Autodesk Inventor part; units mm, degrees
ref_plane "C1_XY" through (0, 0, 0) normal (0, 0, 1) x (1, 0, 0)
ref_plane "C1_YZ" through (0, 0, 0) normal (1, 0, 0) x (0, 1, 0)
ref_plane "C1_ZX" through (0, 0, 0) normal (0, 1, 0) x (0, 0, 1)
sketch "Sketch_63" plane through (0, 0, 0) normal (0, 0, 1) x (1, 0, 0)
  line L0 (-10, -3) -> (-10, -9)
  arc A0 (-10, -9) -> (-9, -10) centre (-9, -9) ccw
  line L1 (-9, -10) -> (9, -10)
  arc A1 (9, -10) -> (10, -9) centre (9, -9) ccw
  line L2 (10, -9) -> (10, -3)
  line L3 (10, -3) -> (8, -3)
  line L4 (8, -3) -> (8, -6)
  line L5 (8, -6) -> (7.0607, -6)
  line L6 (7.0607, -6) -> (4, -2.9393)
  line L7 (4, -2.9393) -> (4, -0.5196)
  line L8 (4, -0.5196) -> (3.7, 0)
  line L9 (3.7, 0) -> (4, 0.5196)
  line L10 (4, 0.5196) -> (4, 2.9393)
  line L11 (4, 2.9393) -> (7.0607, 6)
  line L12 (7.0607, 6) -> (8, 6)
  line L13 (8, 6) -> (8, 3)
  line L14 (8, 3) -> (10, 3)
  line L15 (10, 3) -> (10, 9)
  arc A2 (10, 9) -> (9, 10) centre (9, 9) ccw
  line L16 (9, 10) -> (3, 10)
  line L17 (3, 10) -> (3, 8)
  line L18 (3, 8) -> (6, 8)
  line L19 (6, 8) -> (6, 7.0607)
  line L20 (6, 7.0607) -> (2.9393, 4)
  line L21 (2.9393, 4) -> (0.5196, 4)
  line L22 (0.5196, 4) -> (0, 3.7)
  line L23 (0, 3.7) -> (-0.5196, 4)
  line L24 (-0.5196, 4) -> (-2.9393, 4)
  line L25 (-2.9393, 4) -> (-6, 7.0607)
  line L26 (-6, 7.0607) -> (-6, 8)
  line L27 (-6, 8) -> (-3, 8)
  line L28 (-3, 8) -> (-3, 10)
  line L29 (-3, 10) -> (-9, 10)
  arc A3 (-9, 10) -> (-10, 9) centre (-9, 9) ccw
  line L30 (-10, 9) -> (-10, 3)
  line L31 (-10, 3) -> (-8, 3)
  line L32 (-8, 3) -> (-8, 6)
  line L33 (-8, 6) -> (-7.0607, 6)
  line L34 (-7.0607, 6) -> (-4, 2.9393)
  line L35 (-4, 2.9393) -> (-4, 0.5196)
  line L36 (-4, 0.5196) -> (-3.7, 0)
  line L37 (-3.7, 0) -> (-4, -0.5196)
  line L38 (-4, -0.5196) -> (-4, -2.9393)
  line L39 (-4, -2.9393) -> (-7.0607, -6)
  line L40 (-7.0607, -6) -> (-8, -6)
  line L41 (-8, -6) -> (-8, -3)
  line L42 (-8, -3) -> (-10, -3)
  line L43 (-6, -7.2678) -> (-6, -7.5)
  arc A4 (-6, -7.5) -> (-5.5, -8) centre (-5.5, -7.5) ccw
  line L44 (-5.5, -8) -> (5.5, -8)
  arc A5 (5.5, -8) -> (6, -7.5) centre (5.5, -7.5) ccw
  line L45 (6, -7.5) -> (6, -7.2678)
  arc A6 (6, -7.2678) -> (5.8536, -6.9142) centre (5.5, -7.2678) ccw
  line L46 (5.8536, -6.9142) -> (3.0858, -4.1464)
  arc A7 (3.0858, -4.1464) -> (2.7322, -4) centre (2.7322, -4.5) ccw
  line L47 (2.7322, -4) -> (-2.7322, -4)
  arc A8 (-2.7322, -4) -> (-3.0858, -4.1464) centre (-2.7322, -4.5) ccw
  line L48 (-3.0858, -4.1464) -> (-5.8536, -6.9142)
  arc A9 (-5.8536, -6.9142) -> (-6, -7.2678) centre (-5.5, -7.2678) ccw
extrude "Extrusion1" add sketch "Sketch_63" against normal blind 440
sketch "Sketch2" plane through (0, 0, -440) normal (0, 0, -1) x (-1, 0, 0)
  point P0 (0, 0)
hole "Hole1" at (0, 0, -440) direction (0, 0, 1) diameter 4.2 depth 440
ref_plane "C1_XY" through (0, 0, 0) normal (0, 0, 1) x (1, 0, 0)
ref_plane "C1_YZ" through (0, 0, 0) normal (1, 0, 0) x (0, 1, 0)
ref_plane "C1_ZX" through (0, 0, 0) normal (0, 1, 0) x (0, 0, 1)
thread "Thread1"
thread "Thread2"
properties part number "HFSFB5-2020-440" material "Aluminum 6061"
Geometry: final body of the model. Coordinates: model frame, mm. Round coordinates to 2 decimals unless told otherwise and drop trailing zeros. Put each result on its own line as item: value. Start each with the question number.
Q1. Section A-A on z = -194. Give the number of separate pieces and of enclosed holes in the cut face, and give its area (3 significant figures).
Q2. Line query: probe 1 along Y at (x, z) = (4.75, -345); probe 2 along Y at (x, z) = (0, -267.5); probe 3 along X at (y, z) = (0, -94.5). Output: solid intervals per line, ascending.
Q3. First-contact query: pin 1 (2.5 mm diameter, centred on x = 0, y = 0, fed in from -Z); pin 2 (1.2 mm diameter, centred on y = -1.5, z = -324, fed in from +X). Flat tips, straight axial feed; report the tip coordinate or a pass-through.
Q4. Pull-direction query (X, two-part tool) for faces 1 (the flat face through (0, -8, -217)), 2 (the flat face through (-2.4, 0.1, 0)); classes: +X half, -X half, draft (parallel to the pull), parting line (faces both ways), or undercut.
Ans:
1. separate pieces: 1
1. enclosed holes: 2
1. area: 194 mm2
2. probe 1: y = -10 to -8, -5.81 to -3.69, 3.69 to 5.81, 8 to 10
2. probe 2: y = -10 to -8, -4 to -2.1, 2.1 to 3.7
2. probe 3: x = -3.7 to -2.1, 2.1 to 3.7
3. pin 1: passes through
3. pin 2: stops at x = 4
4. face 1: undercut
4. face 2: draft
